For this review, use the dimensioned drawing (mm, ordinates from the lowest corner) and the shaded views. A direction names the side the tool comes from. Round coordinates to 2 decimals unless told otherwise and drop trailing zeros. Loops run counter-clockwise (first coordinate to the right, second up) from the corner with the lowest first, then second, coordinate; pieces in that order, holes last.
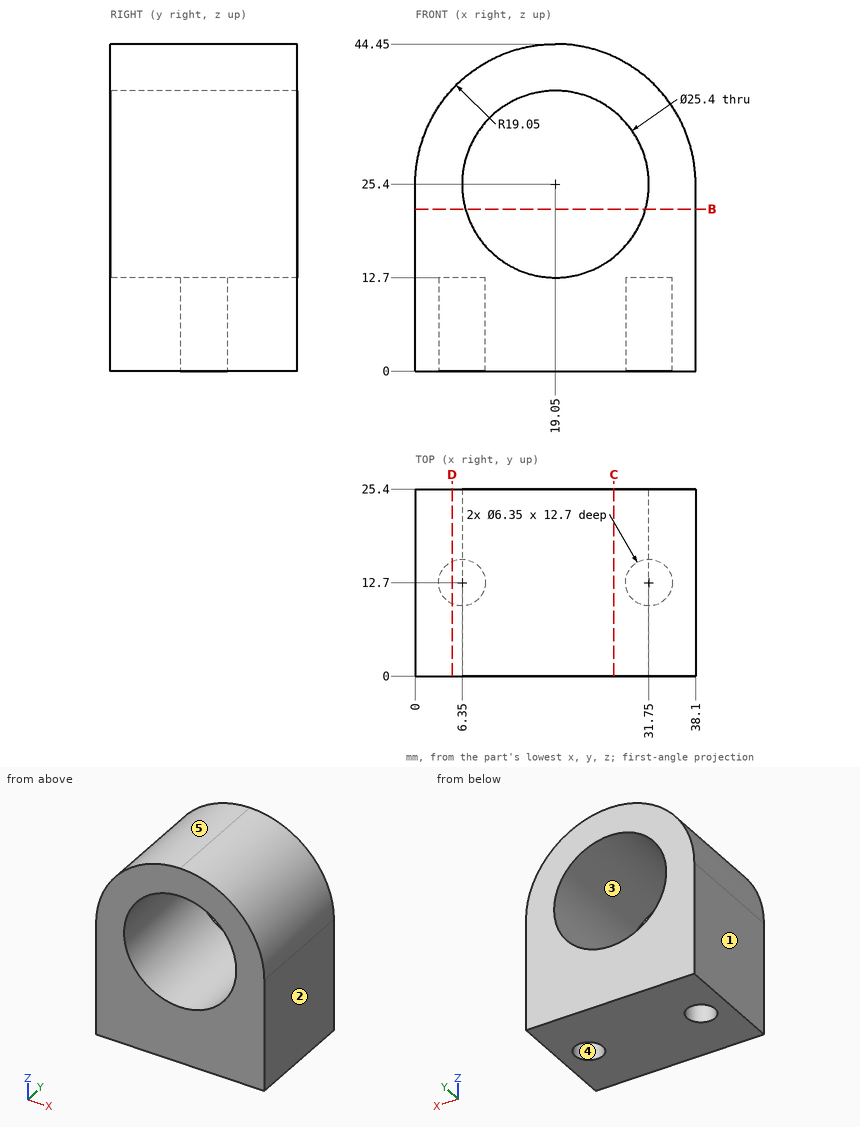
(1) Add section C-C (x = 27). Give the boundary of the cut face in (y, z).
(2) For L1, parallel to Z at x = 19.05, y = 9.75; L2, parallel to Y at x = 31.75, z = 8.25 (3 decimals); L3, parallel to Z at x = 25, y = 17, list the stretches that pass through material, from the lowest coordinate up.
(3) The part is to be moulded in two halves that separate along X. For the marked faces 1, 2 and 3, say which applies: pulls with the +X half, pulls with the -X half, needs draft (parallel to the pull), parting line crosses it, or undercut.
(4) Add section B-B (z = 22). Give the boundary of the cut face in (x, y).
(5) Insertion check: pin 1 Ø6 at (x, y) = (27.5, 22.5) entering from +Z; pin 2 Ø1.9 at (x, y) = (6, 14) entering from -Z; pin 3 Ø2 at (y, z) = (7.5, 36.5) entering from +X; pin 4 Ø20.5 at (x, z) = (19.05, 25.4) entering from -Y. Each pin has a flat end and moves straight along its axis. Give the tip position at first contact, or say it passes through.
(6) Add section D-D (x = 5). Give the boundary of the cut face in (y, z).
(7) For the marked faces 4 and 5, list the 3-axis set-ups (+Z, -Z, +X, -X, +Y, -Y) from which the entire face can be reached by the end or side of a thin tool; tool diameter is ignored.
Outcome:
1. outline: (0, 0) - (25.4, 0) - (25.4, 15.5) - (0, 15.5) - close; (0, 35.3) - (25.4, 35.3) - (25.4, 42.71) - (0, 42.71) - close
2. L1: z = 0 to 12.7, 38.1 to 44.45
2. L2: y = 0 to 9.525, 15.875 to 25.4
2. L3: z = 0 to 14.18, 36.62 to 43.5
3. face 1: pulls with the -X half
3. face 2: pulls with the +X half
3. face 3: undercut
4. outline: (0, 0) - (6.81, 0) - (6.81, 25.4) - (0, 25.4) - close; (31.29, 0) - (38.1, 0) - (38.1, 25.4) - (31.29, 25.4) - close
5. pin 1: stops at z = 43.65
5. pin 2: stops at z = 12.7
5. pin 3: stops at x = 35.2
5. pin 4: passes through
6. outline: (0, 0) - (9.83, 0) - (9.83, 12.7) - (15.57, 12.7) - (15.57, 0) - (25.4, 0) - (25.4, 38.26) - (0, 38.26) - close
7. face 4: -Z
7. face 5: +Z, -X, +Y, -Y
